Could you check a few things on this model? Use its own coordinates, in mm. A direction names the side the tool comes from. Give positions to 0.01 mm unless a question says otherwise; leave off trailing zeros. Loops run counter-clockwise (first coordinate to the right, second up) from the corner with the lowest first, then second, coordinate; pieces in that order, holes last. Notation, with made-up numbers: (8.25, -10.75) - (59.25, -10.75) arc R19 cw to (59.25, 5.25) - close; hole circle Ø6 at (-0.5, 1). An arc over 180 degrees is marked (long way). One line per item, written item: value. Start each with the question number.
Q1. I'm going to push flat-ended pins straight in: P1, Ø1.1, axis at x = 5, y = 3.5, coming from the +Z side; P2, Ø4, axis at x = 31, z = 5, coming from the +Y side; P3, Ø0.8, axis at x = 5, y = 3.5, coming from the +Z side; P4, Ø0.8, axis at y = 3.5, z = -8, coming from the -X side. Where does each tip first touch, or does it pass through?
Q2. I want a section at C-C (z = -19). Please give me the cut outline in (x, y).
Q3. For faces 4 (the face through (0, 3, 0)), 5 (the face through (41, 1, 0)), which set-ups out of +Z, -Z, +X, -X, +Y, -Y let a thin tool reach every point of the face, with its end or its side?
Q4. If I drill on line 1 (X direction, y = 0.8, z = 22); line 2 (Z direction, x = -39, y = 2.05); line 3 (X direction, y = 3.5, z = 12.5), over which ranges is the centre line in solid material (lowest first)? Write a range as from..to.
Q5. I want a section at B-B (x = 4). Please give me the cut outline in (y, z).
Q6. If we mould it in two halves opening along Z, with no side actions, what happens to faces 1 (the face through (-3, 4, 19)), 2 (the face through (37.81, 1.52, 22.16)), 3 (the face through (-1, 1, -24))? For each: released by +Z, released by -Z, zero draft, split by the parting line, or undercut.
Q7. I want a section at A-A (z = 2.5). Please give me the cut outline in (x, y).
Autodesk Inventor part; units mm, degrees
ref_plane "YZ Plane" through (0, 0, 0) normal (1, 0, 0) x (0, 1, 0)
ref_plane "XZ Plane" through (0, 0, 0) normal (0, 1, 0) x (-1, 0, 0)
ref_plane "XY Plane" through (0, 0, 0) normal (0, 0, 1) x (1, 0, 0)
sketch "Boceto1" plane through (0, 0, 0) normal (0, 1, 0) x (-1, 0, 0)
  line L0 (-39, 24) -> (39, 24)
  line L1 (41, 22) -> (41, -22)
  line L2 (39, -24) -> (-39, -24)
  line L3 (-41, -22) -> (-41, 22)
  line L4 (-41, 24) -> (41, -24) construction
  line L5 (41, 24) -> (-41, -24) construction
  arc A0 (39, -24) -> (41, -22) centre (39, -22) ccw
  arc A1 (-41, -22) -> (-39, -24) centre (-39, -22) ccw
  arc A2 (-39, 24) -> (-41, 22) centre (-39, 22) ccw
  arc A3 (41, 22) -> (39, 24) centre (39, 22) ccw
  point P0 (0, 0)
  dimension "d0" = 82
  dimension "d1" = 48
  dimension "d2" = 2
extrude "Extrusión1" add sketch "Boceto1" along normal blind 3
sketch "Boceto2" plane through (0, 3, 0) normal (0, 1, 0) x (1, 0, 0)
  line L0 (38, -21) -> (-38, -21)
  line L1 (-38, -21) -> (-38, 21)
  line L2 (-38, 21) -> (38, 21)
  line L3 (38, 21) -> (38, -21)
  line L4 (38, -21) -> (-38, 21) construction
  line L5 (-38, -21) -> (38, 21) construction
  line L6 (39, 24) -> (-39, 24)
  line L7 (41, -22) -> (41, 22)
  line L8 (35, -18) -> (-35, -18)
  line L9 (-35, -18) -> (-35, 18)
  line L10 (-35, 18) -> (35, 18)
  line L11 (35, 18) -> (35, -18)
  line L12 (35, -18) -> (-35, 18) construction
  line L13 (-35, -18) -> (35, 18) construction
  point P0 (0, 0)
  dimension "d5" = 3
  dimension "d6" = 3
  dimension "d7" = 3
  dimension "d8" = 3
extrude "Extrusión2" add sketch "Boceto2" along normal blind 1
sketch "Boceto3" plane through (0, 0, 0) normal (0, -1, 0) x (1, 0, 0)
  point P0 (-39, 22)
hole "Agujero1" at (-39, 0, 22) direction (0, 1, 0) diameter 2.4 end through all
sketch "Boceto4" plane through (0, 0, 0) normal (0, -1, 0) x (1, 0, 0)
  point P0 (-39, -22)
hole "Agujero2" at (-39, 0, -22) direction (0, 1, 0) diameter 2.4 end through all
sketch "Boceto5" plane through (0, 0, 0) normal (0, -1, 0) x (1, 0, 0)
  point P0 (39, 22)
hole "Agujero3" at (39, 0, 22) direction (0, 1, 0) diameter 2.4 end through all
sketch "Boceto6" plane through (0, 0, 0) normal (0, -1, 0) x (1, 0, 0)
  point P0 (39, -22)
hole "Agujero4" at (39, 0, -22) direction (0, 1, 0) diameter 2.4 end through all
properties part number "Tapa principal" material "Plástico PET"
Worked answers:
1. P1: stops at z = 24
1. P2: stops at y = 3
1. P3: stops at z = 21
1. P4: stops at x = -38
2. outline: (-41, 0) - (41, 0) - (41, 3) - (38, 3) - (38, 4) - (-38, 4) - (-38, 3) - (-41, 3) - close
3. face 4: +Y
3. face 5: +Z, -Z, +X, +Y, -Y
4. line 1: x = -41..-40.2, -37.8..37.8, 40.2..41
4. line 2: z = -24..-23.2, -20.8..20.8, 23.2..24
4. line 3: x = -38..-35, 35..38
5. outline: (0, -24) - (3, -24) - (3, -21) - (4, -21) - (4, -18) - (3, -18) - (3, 18) - (4, 18) - (4, 21) - (3, 21) - (3, 24) - (0, 24) - close
6. face 1: zero draft
6. face 2: undercut
6. face 3: released by -Z
7. outline: (-41, 0) - (41, 0) - (41, 3) - (38, 3) - (38, 4) - (35, 4) - (35, 3) - (-35, 3) - (-35, 4) - (-38, 4) - (-38, 3) - (-41, 3) - close
